Autodesk Inventor part; units mm, degrees
ref_plane "YZ Plane" through (0, 0, 0) normal (1, 0, 0) x (0, 1, 0)
ref_plane "XZ Plane" through (0, 0, 0) normal (0, 1, 0) x (-1, 0, 0)
ref_plane "XY Plane" through (0, 0, 0) normal (0, 0, 1) x (1, 0, 0)
sketch "Náčrt1" plane through (0, 0, 0) normal (0, 1, 0) x (-1, 0, 0)
  line L0 (0, 0) -> (26, 0)
  line L1 (13, -46) -> (0, -46)
  line L2 (0, -46) -> (0, 0)
  line L3 (26, -7.5056) -> (13, 0)
  line L4 (35.4765, -23) -> (0, -23) construction
  arc A0 (26, -13.202) -> (26, -32.798) centre (36, -23) ccw
  line L5 (26, -38.4944) -> (13, -46)
  line L6 (26, -7.5056) -> (26, -13.202)
  line L7 (26, -32.798) -> (26, -38.4944)
  point P0 (13, 0)
  dimension "d15" = -30
  dimension "d17" = 28
  dimension "d18" = 36
  dimension "d19" = 26
  dimension "d20" = 13
  dimension "d21" = 46
  dimension "d22" = 7.5056
extrude "Deska1" add sketch "Náčrt1" along normal blind 3
sketch "Náčrt2" plane through (-3, 0, -46) normal (1, 0, 0) x (0, 1, 0)
  line L0 (0, 46) -> (0, 0)
  line L1 (0, 0) -> (20, 0)
  line L2 (20, 0) -> (20, 46)
  line L3 (20, 46) -> (0, 46)
edge flange "Obruba1" height 20 angle 90 thickness 3 bend radius 3 thickness toward (1, 0, 0) relief tear relief width 3 relief depth 1.5 edges at (0, 3, -23) wall of the first edge with corners at (-3, 0, 0) (-3, 0, -46) (-3, 20, -46) (-3, 20, 0)
bend "Ohyb1"
corner "Roh1"
fillet "Zaoblení rohu1" radius 3 4 edges at (-26, 1.5, -7.5056) (-26, 1.5, -38.4944) (-26, 1.5, -13.202) (-26, 1.5, -32.798)
fillet "Zaoblení rohu2" radius 4 2 edges at (-1.5, 20, -46) (-1.5, 20, 0)
sketch "Náčrt3" plane through (-3, 6, -46) normal (-1, 0, 0) x (0, 0, 1)
  line L0 (42, 14) -> (4, 14)
  line L1 (23, 14) -> (23, 0) construction
  line L2 (46, 0) -> (0, 0) construction
  line L3 (0, -6) -> (46, -6) construction
  point P0 (41, 9)
  point P1 (5, 9)
  dimension "d25" = 36
  dimension "d26" = 15
hole "Díra1" at (-3, 15, -5) at (-3, 15, -41) direction (1, 0, 0) diameter 4.5 end through all
sketch "Náčrt4" plane through (0, 3, 0) normal (0, 1, 0) x (1, 0, 0)
  line L0 (-21, 13.5) -> (-17, 13.5) construction
  line L1 (-21, 11.25) -> (-17, 11.25)
  line L2 (-17, 15.75) -> (-21, 15.75)
  arc A0 (-21, 15.75) -> (-21, 11.25) centre (-21, 13.5) ccw
  arc A1 (-17, 11.25) -> (-17, 15.75) centre (-17, 13.5) ccw
  arc A2 (-26, 13.202) -> (-26, 32.798) centre (-36, 23) ccw
  line L3 (-22, 23) -> (-6, 23) construction
  line L4 (-6, 0) -> (-6, 46) construction
  line L5 (-21, 32.5) -> (-17, 32.5) construction
  line L6 (-21, 34.75) -> (-17, 34.75)
  line L7 (-17, 30.25) -> (-21, 30.25)
  arc A3 (-21, 34.75) -> (-21, 30.25) centre (-21, 32.5) ccw
  arc A4 (-17, 30.25) -> (-17, 34.75) centre (-17, 32.5) ccw
  line L8 (-6, 0) -> (-13, 0) construction
  line L9 (-26, 9.2376) -> (-26, 13.202) construction
  point P0 (0, 0)
  point P1 (-19, 13.5)
  point P2 (-19, 32.5)
  point P3 (-19, 32.5)
  dimension "d36" = 4
  dimension "d37" = 4.5
  dimension "d40" = 19
  dimension "d41" = 5
extrude "Vysunutí1" cut sketch "Náčrt4" against normal up to next
equation "\"d32\" = Tloušťka"
equation "\"d3\" = Tloušťka"
equation "\"d4\" = ŠířkaVýštipu"
equation "\"d5\" = HloubkaVýštipu"
equation "\"d6\" = MinimálníZbytek"
equation "\"d7\" = PřechodovýPoloměr"
equation "\"d10\" = PoloměrOhybu"
equation "\"d11\" = VelikostRohovéhoVýštipu"
equation "\"d12\" = VelikostMezery"
equation "\"d13\" = VelikostJacobihoPoloměru"
equation "\"PoloměrOhybu\" = Tloušťka"
equation "\"ŠířkaVýštipu\" = Tloušťka"
equation "\"HloubkaVýštipu\" = 0.5 * Tloušťka"
equation "\"VelikostRohovéhoVýštipu\" = 4 * Tloušťka"
equation "\"MinimálníZbytek\" = 2 * Tloušťka"
equation "\"PřechodovýPoloměr\" = PoloměrOhybu"
equation "\"VelikostJacobihoPoloměru\" = PoloměrOhybu"
equation "\"VelikostMezery\" = Tloušťka"
properties part number "drzak_valce2" material "Železo, kujné"
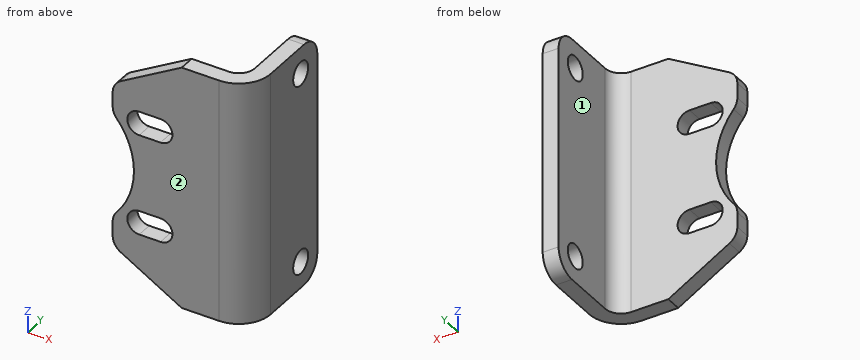
Work out the finished part from the listing and answer in its coordinate system (mm). Face numbers are marked on the shaded views. A direction names the side the tool comes from. Round coordinates to 2 decimals unless told otherwise and drop trailing zeros. Write each loop counter-clockwise with the first axis right and the second up, starting at its lowest first coordinate (ties: lowest second). Pieces come first, ordered by that corner, then holes. Notation, with made-up numbers: (33.25, -38.75) - (62.25, -38.75) arc R13 ccw to (62.25, -15.75) - close; hole circle Ø3 at (-32, 33). An arc over 180 degrees is marked (long way). Return JSON: item names as keys, results as strings. Group by question number.
Q1. The part is cut by section A-A on y = 15. Write down the section's boundary in (x, z).
Q2. For the marked faces 1 and 2, determine the directions among +Z, -Z, +X, -X, +Y, -Y from which every point of the face is accessible in a straight line to the end or side of a thin tool.
Q3. The part is cut by section B-B on z = -41. Write down the section's boundary in (x, y), then the cut area to 3 significant figures.
Q4. Each of these flat-tipped pins is pushed along its axis until it touches: pin 1 Ø0.9 at (x, y) = (-18.5, 1.5) entering from -Z; pin 2 Ø3.5 at (x, y) = (-18.5, 2) entering from +Z; pin 3 Ø10 at (y, z) = (17, -29) entering from +X; pin 4 Ø5 at (y, z) = (17, -39.5) entering from -X. Where does it stop, or does it pass through?
Q5. Find the intervals of material crossed by L1, parallel to Z at x = -1.3, y = 15; L2, parallel to X at y = 8, z = -32.5; L3, parallel to Y at x = -9.5, z = -17, in increasing order.
Q6. The part is cut by section D-D on z = -32.5. Write down the section's boundary in (x, y).
Q7. The part is cut by section C-C on x = -19.5. Write down the section's boundary in (y, z), then the cut area to 3 significant figures.
Solved:
{
 "1": {"outline": "(-3, -46) - (0, -46) - (0, -43.25) - (-3, -43.25) - close; (-3, -38.75) - (0, -38.75) - (0, -7.25) - (-3, -7.25) - close; (-3, -2.75) - (0, -2.75) - (0, 0) - (-3, 0) - close"},
 "2": {"face 1": "+Z, -Z, -X, +Y", "face 2": "+Z, -Z, +X, -X, -Y"},
 "3": {"outline": "(-21.66, 0) - (-6, 0) arc R6 ccw to (0, 6) - (0, 12.75) - (-3, 12.75) - (-3, 6) arc R3 cw to (-6, 3) - (-21.66, 3) - close; (-3, 17.25) - (0, 17.25) - (0, 20) - (-3, 20) - close", "area": "96.7 mm²"},
 "4": {"pin 1": "z = -43.08", "pin 2": "z = -2.17", "pin 3": "x = 0", "pin 4": "x = -3"},
 "5": {"L1": "-46 to -43.25, -38.75 to -7.25, -2.75 to 0", "L2": "-3 to 0", "L3": "0 to 3"},
 "6": {"outline": "(-25.62, 0) - (-23.25, 0) - (-23.25, 3) - (-25.62, 3) - close; (-14.75, 0) - (-6, 0) arc R6 ccw to (0, 6) - (0, 20) - (-3, 20) - (-3, 6) arc R3 cw to (-6, 3) - (-14.75, 3) - close"},
 "7": {"outline": "(0, -42.25) - (3, -42.25) - (3, -34.75) - (0, -34.75) - close; (0, -30.25) - (3, -30.25) - (3, -15.75) - (0, -15.75) - close; (0, -11.25) - (3, -11.25) - (3, -3.75) - (0, -3.75) - close", "area": "88.5 mm²"}
}
